```python
from build123d import *

# Parameters (mm, degrees)
SKETCH1_R           = 1.6
BOSS_EXTRUDE1_DEPTH = 4
SKETCH2_R           = 6
SKETCH2_R_2         = 1.6
BOSS_EXTRUDE2_DEPTH = 2
CHAMFER1_SIZE       = 1.5


with BuildPart() as part:
    # Sketch1 → Boss-Extrude1 (new body)
    with BuildSketch(Plane(origin=(0, 0, 0), x_dir=(1, 0, 0), z_dir=(0, 1, 0))):
        with BuildLine():
            Line((-6, 0), (-6, 8))
            ThreePointArc((-6, 8), (0, 14), (6, 8))
            Line((6, 8), (6, 0))
            ThreePointArc((6, 0), (0, -6), (-6, 0))
        make_face()
        with Locations(Location((0, 0, 0), (0, 0, 270))):
            Circle(SKETCH1_R, mode=Mode.SUBTRACT)
    extrude(amount=BOSS_EXTRUDE1_DEPTH)

    # Sketch2 → Boss-Extrude2 (add)
    with BuildSketch(Plane(origin=(0, 4, 0), x_dir=(1, 0, 0), z_dir=(0, 1, 0))):
        Circle(SKETCH2_R)
        with Locations(Location((0, 0, 0), (0, 0, 270))):
            Circle(SKETCH2_R_2, mode=Mode.SUBTRACT)
    extrude(amount=BOSS_EXTRUDE2_DEPTH)

    # Chamfer1
    # the kernel refuses this chamfer: 1.5 mm, written as the material it takes off along each edge
    with BuildSketch(Plane(origin=(0, 6, 0), x_dir=(1, 0, 0), z_dir=(0, 0, 1))) as chamfer1_piece_1:
        Polygon((6, -CHAMFER1_SIZE), (6 - CHAMFER1_SIZE, 0), (6, 0), align=None)
    revolve(axis=Axis((0, 6, 0), (0, 1, 0)), mode=Mode.SUBTRACT)
    with BuildSketch(Plane(origin=(6, 4, -8), x_dir=(0.0274958766105862, -0.9996219169112968, 0), z_dir=(0, 0, 1))) as chamfer1_piece_2_section:
        Polygon((CHAMFER1_SIZE * 0.999621916911, -CHAMFER1_SIZE * 0.0274958766106), (-CHAMFER1_SIZE * 0.0274958766106, -CHAMFER1_SIZE * 0.999621916911), (0, 0), align=None)
    chamfer1_piece_2 = extrude(amount=11.857524482, mode=Mode.PRIVATE)
    chamfer1_piece_2 = chamfer1_piece_2 - Plane(origin=(0, 3.415911746, 0), x_dir=(1, 0, 0), z_dir=(0, -1, 0)) * Cylinder(6, 30, mode=Mode.PRIVATE)
    add(chamfer1_piece_2, mode=Mode.SUBTRACT)
    with BuildSketch(Plane(origin=(0, 4, -8), x_dir=(-1, 0, 0), z_dir=(0, 0, 1))) as chamfer1_piece_3:
        Polygon((6, CHAMFER1_SIZE), (6 - CHAMFER1_SIZE, 0), (6, 0), align=None)
    revolve(axis=Axis((0, 4, -8), (0, -1, 0)), revolution_arc=180, mode=Mode.SUBTRACT)
    with BuildSketch(Plane(origin=(-6, 4, 3.857524482), x_dir=(0.9996219169112969, 0.02749587661058621, 0), z_dir=(0, 0, -1))) as chamfer1_piece_4_section:
        Polygon((CHAMFER1_SIZE * 0.999621916911, CHAMFER1_SIZE * 0.0274958766106), (-CHAMFER1_SIZE * 0.0274958766106, CHAMFER1_SIZE * 0.999621916911), (0, 0), align=None)
    chamfer1_piece_4 = extrude(amount=11.857524482, mode=Mode.PRIVATE)
    chamfer1_piece_4 = chamfer1_piece_4 - Plane(origin=(0, 3.415911747, 0), x_dir=(1, 0, 0), z_dir=(0, -1, 0)) * Cylinder(6, 30, mode=Mode.PRIVATE)
    add(chamfer1_piece_4, mode=Mode.SUBTRACT)


solid = part.part
```
Design review of the part built by this model. Coordinates are the model's own, in mm. A direction names the side the tool comes from. Coordinates: 2 decimals unless noted, no trailing zeros. Write each loop counter-clockwise with the first axis right and the second up, starting at its lowest first coordinate (ties: lowest second). Pieces come first, ordered by that corner, then holes.
1) To check wall thickness, follow L1, parallel to X at y = 4.45, z = 0; L2, parallel to Z at x = 1, y = 3.7; L3, parallel to Z at x = -0.75, y = 4.3. State the ranges of each line that lie inside material, in increasing order.
2) Add section A-A (x = 0). Write out the cut boundary in (y, z), plus the area to 3 significant figures.
3) Mouldability with a two-part tool opening along X and no side actions: class faces 1 (the flat face through (0, 6, 2)), 2 (the conical face through (-0.1, 3.8, -12.7)), 3 (the flat face through (-6, 1, -4)), 4 (the cylindrical face through (-0.97, 2.96, -1.27)) as +X half, -X half, draft (parallel to the pull), parting line (faces both ways), or undercut.
4) Machinability: for faces 5 (the flat face through (-5.2, 3.3, -4.8)), 6 (the flat face through (5.3, 3.2, -4.9)), 7 (the cylindrical face through (-1.301, 2.718, 5.857)), which of the approach directions +Z, -Z, +X, -X, +Y, -Y give a long, thin tool a straight path to every point of the face, cutting with its end or side? Answer none if there is none.
5) Add section C-C (y = 4.9). Write out the cut boundary in (x, z), plus the area to 3 significant figures.
6) Insertion check: pin 1 (1.9 mm diameter, centred on x = 0, z = 0, fed in from +Y); pin 2 (3 mm diameter, centred on x = -2.5, y = 3.5, fed in from +Z); pin 3 (1 mm diameter, centred on x = -2, y = 5, fed in from -Z). Each pin has a flat end and moves straight along its axis. Give the tip position at first contact, or say it passes through.
7) Add section B-B (y = 2). Write out the cut boundary in (x, z).
Check result:
1. L1: x = -6 to -1.6, 1.6 to 6
1. L2: z = -12.69 to -1.25, 1.25 to 5.92
1. L3: z = -5.95 to -1.41, 1.41 to 5.95
2. outline: (0, -14) - (2.5, -14) - (4, -12.5) - (4, -6) - (4.5, -6) - (6, -4.5) - (6, -1.6) - (0, -1.6) - close; (0, 1.6) - (6, 1.6) - (6, 4.5) - (4.5, 6) - (0, 6) - close
2. area: 81.4 mm2
3. face 1: draft
3. face 2: parting line
3. face 3: -X half
3. face 4: undercut
4. face 5: -Z, -X, +Y
4. face 6: -Z, +X, +Y
4. face 7: +Y
5. outline: circle Ø11.2 at (0, 0); hole circle Ø3.2 at (0, 0)
5. area: 90.5 mm2
6. pin 1: passes through
6. pin 2: stops at z = 5.92
6. pin 3: stops at z = -5.68
7. outline: (-6, -8) arc R6 ccw to (6, -8) - (6, 0) arc R6 ccw to (-6, 0) - close; hole circle Ø3.2 at (0, 0)
